from build123d import *

# Parameters (mm, degrees)
SALIENTE_EXTRUIR1_DEPTH = 112
VACIADO1_START          = 5
VACIADO1_DEPTH          = 102
REDONDEO1_R             = 5
CROQUIS2_W              = 71.4
CROQUIS2_H              = 27
CORTAR_EXTRUIR1_DEPTH   = 10
CORTAR_EXTRUIR2_DEPTH   = 1
CORTAR_EXTRUIR9_DEPTH   = 4
CROQUIS5_R              = 1
CROQUIS5_R_2            = 1.5
CORTAR_EXTRUIR3_DEPTH   = 6
CROQUIS6_W              = 51.5
CROQUIS6_H              = 100.8
CORTAR_EXTRUIR4_DEPTH   = 3.4
CROQUIS7_W              = 7.2
CROQUIS7_H              = 1.2
CORTAR_EXTRUIR6_DEPTH   = 119.765525301
CROQUIS14_W             = 11
CROQUIS14_H             = 9
CORTAR_EXTRUIR11_DEPTH  = 3
REDONDEO2_R             = 0.3


# Read off the part's stored shape, not the designer's step: Vaciado1
with BuildPart() as part:
    # Croquis1 → Saliente-Extruir1 (new body)
    with BuildSketch(Plane.XY):
        Polygon((-32.5, 0), (0, 40), (32.5, 40), (32.5, -40), (-32.5, -40), align=None)
    extrude(amount=SALIENTE_EXTRUIR1_DEPTH)

    # Vaciado1 outline → Vaciado1 (cut)
    with BuildSketch(Plane.XY.offset(VACIADO1_START)):
        Polygon((32.5, 35), (6.245264064, 35), (-27.5, -6.532632694), (-27.5, -32), (32.5, -32), align=None)
    extrude(amount=VACIADO1_DEPTH, mode=Mode.SUBTRACT)

    # Redondeo1
    redondeo1_edges = [part.edges().sort_by_distance(p)[0] for p in [
        (-16.25, 20, 112),
        (-32.5, -20, 112),
        (0, -40, 112),
        (32.5, 0, 112),
        (0, -40, 0),
        (-32.5, -20, 0),
        (-16.25, 20, 0),
        (16.25, 40, 0),
        (32.5, 0, 0),
        (16.25, 40, 112),
        (32.5, -40, 56),
        (-32.5, -40, 56),
        (-32.5, 0, 56),
        (0, 40, 56),
    ]]
    fillet(redondeo1_edges, radius=REDONDEO1_R - 0.0001)  # a hair under: the kernel refuses the full size

    # Croquis2 → Cortar-Extruir1 (cut)
    with BuildSketch(Plane(origin=(-19.576470588, 15.905882353, 0), x_dir=(0, 0, 1), z_dir=(-0.7761140001162655, 0.6305926250944658, 0))):
        with Locations((56, 5.275149845)):
            Rectangle(CROQUIS2_W, CROQUIS2_H)
    extrude(amount=-CORTAR_EXTRUIR1_DEPTH, mode=Mode.SUBTRACT)

    # Croquis3 → Cortar-Extruir2 (cut)
    with BuildSketch(Plane(origin=(-13.367558587, 10.861141352, 0), x_dir=(0, 0, -1), z_dir=(0.7761140001162655, -0.6305926250944659, 0))):
        with BuildLine():
            Line((-97, -11.224850155), (-15, -11.224850155))
            ThreePointArc((-15, -11.224850155), (-12.878679656, -10.346170499), (-12, -8.224850155))
            Line((-12, -8.224850155), (-12, 18.775149845))
            ThreePointArc((-12, 18.775149845), (-12.878679656, 20.896470188), (-15, 21.775149845))
            Line((-15, 21.775149845), (-97, 21.775149845))
            ThreePointArc((-97, 21.775149845), (-99.121320344, 20.896470188), (-100, 18.775149845))
            Line((-100, 18.775149845), (-100, -8.224850155))
            ThreePointArc((-100, -8.224850155), (-99.121320344, -10.346170499), (-97, -11.224850155))
        make_face()
    extrude(amount=-CORTAR_EXTRUIR2_DEPTH, mode=Mode.SUBTRACT)

    # Croquis10 → Cortar-Extruir9 (cut)
    with BuildSketch(Plane(origin=(-14.143672587, 11.491733977, 0), x_dir=(0, 0, -1), z_dir=(0.7761140001162654, -0.630592625094466, 0))):
        Polygon((-91.7, -2.724850155), (-91.7, 13.275149845), (-100, 9.275149845), (-100, 1.275149845), align=None)
    extrude(amount=-CORTAR_EXTRUIR9_DEPTH, mode=Mode.SUBTRACT)

    # Croquis5 → Cortar-Extruir3 (cut)
    with BuildSketch(Plane(origin=(-14.143672587, 11.491733977, 0), x_dir=(0, 0, -1), z_dir=(0.7761140001162655, -0.6305926250944659, 0))):
        with Locations(Location((-96.5, 18.275149845, 0), (0, 0, 90))):
            Circle(CROQUIS5_R)
        with Locations(Location((-96.5, -7.724850155, 0), (0, 0, 90))):
            Circle(CROQUIS5_R_2)
        with Locations(Location((-15.5, -7.724850155, 0), (0, 0, 90))):
            Circle(CROQUIS5_R)
        with Locations(Location((-15.5, 18.275149845, 0), (0, 0, 90))):
            Circle(CROQUIS5_R_2)
    extrude(amount=-CORTAR_EXTRUIR3_DEPTH, mode=Mode.SUBTRACT)

    # Croquis6 → Cortar-Extruir4 (cut)
    with BuildSketch(Plane(origin=(0, -32, 0), x_dir=(1, 0, 0), z_dir=(0, 1, 0))):
        with Locations((2.5, -56)):
            Rectangle(CROQUIS6_W, CROQUIS6_H)
    extrude(amount=-CORTAR_EXTRUIR4_DEPTH, mode=Mode.SUBTRACT)

    # Croquis7 → Cortar-Extruir6 (cut, through all)
    with BuildSketch(Plane.XY.offset(5)):
        Polygon((-2.7, -18), (4.5, -18), (5, -17.1), (5, -15), (-3.2, -15), (-3.2, -17.1), align=None)
        with Locations((0.9, -18.6)):
            Rectangle(CROQUIS7_W, CROQUIS7_H)
    extrude(amount=-CORTAR_EXTRUIR6_DEPTH, mode=Mode.SUBTRACT)

    # Croquis14 → Cortar-Extruir11 (cut)
    with BuildSketch(Plane(origin=(0, 0, 0), x_dir=(-1, 0, 0), z_dir=(0, 0, -1))):
        with Locations((-0.9, -17.1)):
            Rectangle(CROQUIS14_W, CROQUIS14_H)
    extrude(amount=-CORTAR_EXTRUIR11_DEPTH, mode=Mode.SUBTRACT)

    # Redondeo2
    redondeo2_edges = [part.edges().sort_by_distance(p)[0] for p in [
        (-2.95, -17.55, 5),
        (-3.2, -16.05, 5),
        (0.9, -15, 5),
        (-2.7, -18.6, 5),
        (0.9, -19.2, 5),
        (4.5, -18.6, 5),
        (4.75, -17.55, 5),
        (5, -16.05, 5),
        (-2.7, -19.2, 4),
        (-2.7, -18, 4),
        (-2.7, -18.6, 3),
        (4.5, -19.2, 4),
        (4.5, -18, 4),
        (5, -17.1, 4),
        (5, -15, 4),
        (-3.2, -15, 4),
        (-3.2, -17.1, 4),
        (-3.2, -16.05, 3),
        (-2.95, -17.55, 3),
        (0.9, -15, 3),
        (6.4, -17.1, 3),
        (6.4, -21.6, 1.5),
        (0.9, -12.6, 3),
        (6.4, -12.6, 1.5),
        (-4.6, -17.1, 3),
        (-4.6, -12.6, 1.5),
        (0.9, -21.6, 3),
        (-4.6, -21.6, 1.5),
        (5, -16.05, 3),
        (4.75, -17.55, 3),
        (4.5, -18.6, 3),
        (0.9, -19.2, 3),
        (6.4, -17.1, 0),
        (0.9, -21.6, 0),
        (-4.6, -17.1, 0),
        (0.9, -12.6, 0),
    ]]
    fillet(redondeo2_edges, radius=REDONDEO2_R)


solid = part.part
Verification items for the finished model (mm, model axes). A direction names the side the tool comes from. Round coordinates to 2 decimals unless told otherwise and drop trailing zeros. Loops run counter-clockwise (first coordinate to the right, second up) from the corner with the lowest first, then second, coordinate; pieces in that order, holes last. Notation, with made-up numbers: M 30.25,65 L 85.25,65 A27 cw 85.25,86 Z; hole C 46,61 d6. An arc over 180 degrees is marked long. Write each question's results on one line, items separated by ' | '.
1) Section check B-B on z = 79. Record the boundary of the cut face in (x, y), then the cut area to 3 significant figures.
Checks:
outline: M -32.5,-35 A5 ccw -27.5,-40 L 27.5,-40 A5 ccw 32.5,-35 L 32.5,-32 L 28.25,-32 L 28.25,-35.4 L -23.25,-35.4 L -23.25,-32 L -27.5,-32 L -27.5,-6.53 L -20.45,2.15 L -21.22,2.78 L -19.33,5.11 L -24.76,9.52 L -31.38,1.38 A5 ccw -32.5,-1.78 Z; M -7.74,30.48 L -2.3,26.06 L -0.41,28.39 L 0.36,27.76 L 6.25,35 L 32.5,35 L 32.5,40 L 2.38,40 A5 ccw -1.5,38.15 Z | area: 822 mm2
2) Scan lines: L1, parallel to Y at x = 27, z = 57; L2, parallel to Z at x = 9, y = -5; L3, parallel to X at y = -14, z = 73. Record each from-to range of solid material in increasing order. Write a range as from..to.
Checks:
L1: y = -40..-35.4, 35..40 | L2: z = 0..5, 107..112 | L3: x = -32.5..-27.5
3) Access from +Z, -Z, +X, -X, +Y, -Y to the whole of each face (thin tool, end or side, straight path). Record for faces 1 (the flat face through (6.4, -17, 1)), 2 (the flat face through (-8.55, 21.51, 95.79)), 3 (the flat face through (-11, 15, 12)).
Checks:
face 1: -Z | face 2: none | face 3: +X
4) Gauge pin test, flat ends, axial feed: P1, Ø1.9, axis at x = 2.5, z = 1, coming from the -Y side; P2, Ø11, axis at x = -19, y = 21.5, coming from the -Z side; P3, Ø1.2, axis at x = 0.5, z = 1.5, coming from the +Y side. Record the tip position at first contact, or that the pin passes through.
Checks:
P1: stops at y = -38.96 | P2: stops at z = 0.72 | P3: stops at y = 38.69
5) Mould release check, pull along X, two halves, no side actions. Record for faces 4 (the cylindrical face through (-0.588, 27.372, 12.855)), 5 (the cylindrical face through (-32.204, -0.08, 56.714)), 6 (the flat face through (1, -12.6, 1)), 7 (the flat face through (-16.11, 12.19, 95.91)): released by +X, released by -X, zero draft, split by the parting line, or undercut.
Checks:
face 4: undercut | face 5: released by -X | face 6: undercut | face 7: released by +X
6) Section check A-A on x = 14.5. Record the boundary of the cut face in (y, z).
Checks:
outline: M -40,5 A5 ccw -35,0 L 35,0 A5 ccw 40,5 L 40,107 A5 ccw 35,112 L -35,112 A5 ccw -40,107 Z; hole M -35.4,5.6 L -32,5.6 L -32,5 L 35,5 L 35,107 L -32,107 L -32,106.4 L -35.4,106.4 Z
